Answer from the drawing. Dimensions are ordinates in mm from the lowest x, y and z of the part. Give positions to 0.01 mm unless a question says otherwise; leave off trailing zeros. Loops run counter-clockwise (first coordinate to the right, second up) from the corner with the lowest first, then second, coordinate; pieces in that order, holes last. Notation, with made-up numbers: (74, 51.5) - (117, 51.5) arc R18 ccw to (117, 69.5) - close; hole circle Ø1 at (34, 42.5). An arc over 180 degrees is marked (long way). Put each result on its own line as item: value. Start each with the question number.
1. A cutting plane is placed at C-C, the plane x = 34.5. Determine the outline of the cut face in (y, z).
2. A cutting plane is placed at A-A, the plane y = 38.5. Determine the outline of the cut face in (x, z).
3. A cutting plane is placed at D-D, the plane z = 137. Determine the outline of the cut face in (x, y).
4. Given pin 1 Ø1 at (x, y) = (81.5, 14) entering from -Z; pin 2 Ø6 at (x, z) = (258, 133) entering from +Y; pin 3 Ø1.5 at (y, z) = (87, 106.5) entering from -X, each flat-ended and moving along its own axis, determine where each tip first touches the part or whether it passes through.
5. Consider L1, parallel to Y at x = 206.5, z = 151; L2, parallel to Z at x = 83, y = 37. Determine where each line is inside the solid, lowest interval first. Write a range as from..to.
6. A cutting plane is placed at B-B, the plane x = 156. Determine the outline of the cut face in (y, z).
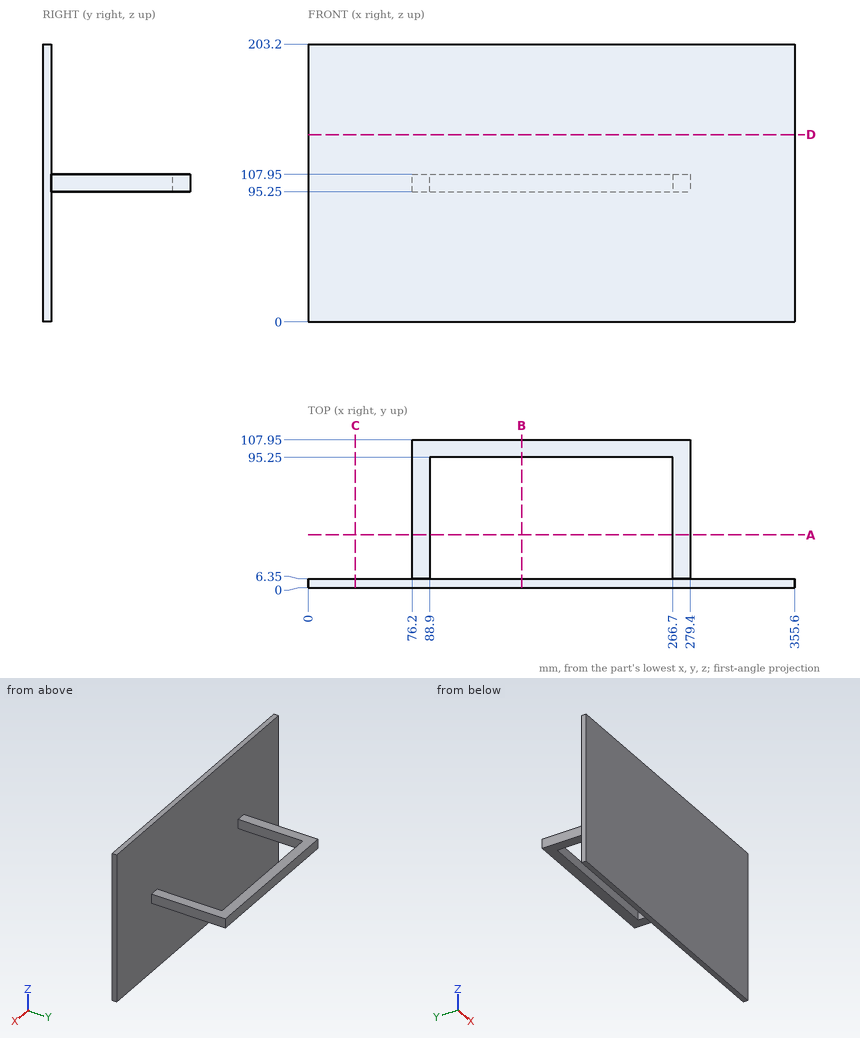
Return value:
1. outline: (0, 0) - (6.35, 0) - (6.35, 203.2) - (0, 203.2) - close
2. outline: (76.2, 95.25) - (88.9, 95.25) - (88.9, 107.95) - (76.2, 107.95) - close; (266.7, 95.25) - (279.4, 95.25) - (279.4, 107.95) - (266.7, 107.95) - close
3. outline: (0, 0) - (355.6, 0) - (355.6, 6.35) - (0, 6.35) - close
4. pin 1: stops at z = 95.25
4. pin 2: stops at y = 6.35
4. pin 3: stops at x = 76.2
5. L1: y = 0..6.35
5. L2: z = 95.25..107.95
6. outline: (0, 0) - (6.35, 0) - (6.35, 203.2) - (0, 203.2) - close; (95.25, 95.25) - (107.95, 95.25) - (107.95, 107.95) - (95.25, 107.95) - close
